CAD build for the part. Positions are in the model's coordinates, mm. Face numbers are marked on the shaded views. Round coordinates to 2 decimals unless told otherwise and drop trailing zeros. Write each loop counter-clockwise with the first axis right and the second up, starting at its lowest first coordinate (ties: lowest second). Pieces come first, ordered by that corner, then holes. Notation, with made-up numbers: (43.25, -11.5) -> (49.25, -11.5) arc R34 cw to (49.25, 23.5) -> close; hole circle Ø11 at (75.5, -37). An arc over 180 degrees is marked (long way). Answer in a Markdown table with one row per item. Add a question column.
```python
from build123d import *

# Parameters (mm, degrees)
F1_DEPTH = 11
F3_DEPTH = 1.5


with BuildPart() as f1:
    # F0 (on Top) → F1 (new body)
    with BuildSketch(Plane.XY):
        with BuildLine():
            ThreePointArc((-67.1, 20.6), (-67.312132, 20.512132), (-67.4, 20.3))
            Line((-67.4, 20.3), (-67.4, 0.3))
            ThreePointArc((-67.4, 0.3), (-67.312132, 0.087868), (-67.1, 0))
            Line((-67.1, 0), (-64.043352, 0))
            ThreePointArc((-64.043352, 0), (-63.77146, -0.173215), (-63.813539, -0.492836))
            Line((-63.813539, -0.492836), (-68.349465, -5.898542))
            ThreePointArc((-68.349465, -5.898542), (-68.41851, -6.117525), (-68.312488, -6.321192))
            Line((-68.312488, -6.321192), (-67.469839, -7.028258))
            ThreePointArc((-67.469839, -7.028258), (-67.250856, -7.097303), (-67.047189, -6.991281))
            Line((-67.047189, -6.991281), (-61.270729, -0.107164))
            ThreePointArc((-61.270729, -0.107164), (-61.167701, -0.028108), (-61.040915, 0))
            Line((-61.040915, 0), (-49.043352, 0))
            ThreePointArc((-49.043352, 0), (-48.77146, -0.173215), (-48.813539, -0.492836))
            Line((-48.813539, -0.492836), (-53.349465, -5.898542))
            ThreePointArc((-53.349465, -5.898542), (-53.41851, -6.117525), (-53.312488, -6.321192))
            Line((-53.312488, -6.321192), (-52.469839, -7.028258))
            ThreePointArc((-52.469839, -7.028258), (-52.250856, -7.097303), (-52.047189, -6.991281))
            Line((-52.047189, -6.991281), (-46.270729, -0.107164))
            ThreePointArc((-46.270729, -0.107164), (-46.167701, -0.028108), (-46.040915, 0))
            Line((-46.040915, 0), (-34.043352, 0))
            ThreePointArc((-34.043352, 0), (-33.77146, -0.173215), (-33.813539, -0.492836))
            Line((-33.813539, -0.492836), (-38.349465, -5.898542))
            ThreePointArc((-38.349465, -5.898542), (-38.41851, -6.117525), (-38.312488, -6.321192))
            Line((-38.312488, -6.321192), (-37.469839, -7.028258))
            ThreePointArc((-37.469839, -7.028258), (-37.250856, -7.097303), (-37.047189, -6.991281))
            Line((-37.047189, -6.991281), (-31.270729, -0.107164))
            ThreePointArc((-31.270729, -0.107164), (-31.167701, -0.028108), (-31.040915, 0))
            Line((-31.040915, 0), (-19.043352, 0))
            ThreePointArc((-19.043352, 0), (-18.77146, -0.173215), (-18.813539, -0.492836))
            Line((-18.813539, -0.492836), (-23.349465, -5.898542))
            ThreePointArc((-23.349465, -5.898542), (-23.41851, -6.117525), (-23.312488, -6.321192))
            Line((-23.312488, -6.321192), (-22.469839, -7.028258))
            ThreePointArc((-22.469839, -7.028258), (-22.250856, -7.097303), (-22.047189, -6.991281))
            Line((-22.047189, -6.991281), (-16.270729, -0.107164))
            ThreePointArc((-16.270729, -0.107164), (-16.167701, -0.028108), (-16.040915, 0))
            Line((-16.040915, 0), (-4.043352, 0))
            ThreePointArc((-4.043352, 0), (-3.77146, -0.173215), (-3.813539, -0.492836))
            Line((-3.813539, -0.492836), (-8.349465, -5.898542))
            ThreePointArc((-8.349465, -5.898542), (-8.41851, -6.117525), (-8.312488, -6.321192))
            Line((-8.312488, -6.321192), (-7.469839, -7.028258))
            ThreePointArc((-7.469839, -7.028258), (-7.250856, -7.097303), (-7.047189, -6.991281))
            Line((-7.047189, -6.991281), (-1.270729, -0.107164))
            ThreePointArc((-1.270729, -0.107164), (-1.167701, -0.028108), (-1.040915, 0))
            Line((-1.040915, 0), (10.956648, 0))
            ThreePointArc((10.956648, 0), (11.22854, -0.173215), (11.186461, -0.492836))
            Line((11.186461, -0.492836), (6.650535, -5.898542))
            ThreePointArc((6.650535, -5.898542), (6.58149, -6.117525), (6.687512, -6.321192))
            Line((6.687512, -6.321192), (7.530161, -7.028258))
            ThreePointArc((7.530161, -7.028258), (7.749144, -7.097303), (7.952811, -6.991281))
            Line((7.952811, -6.991281), (13.729271, -0.107164))
            ThreePointArc((13.729271, -0.107164), (13.832299, -0.028108), (13.959085, 0))
            Line((13.959085, 0), (20.524052, 0))
            ThreePointArc((20.524052, 0), (20.795944, -0.173215), (20.753865, -0.492836))
            Line((20.753865, -0.492836), (19.063644, -2.507164))
            ThreePointArc((19.063644, -2.507164), (19.021565, -2.826785), (19.293457, -3))
            Line((19.293457, -3), (21.121027, -3))
            ThreePointArc((21.121027, -3), (21.247813, -2.971892), (21.35084, -2.892836))
            Line((21.35084, -2.892836), (24.436221, 0.784177))
            ThreePointArc((24.436221, 0.784177), (24.539249, 0.863233), (24.666034, 0.891341))
            Line((24.666034, 0.891341), (25.188197, 0.891341))
            ThreePointArc((25.188197, 0.891341), (25.46009, 0.718126), (25.418011, 0.398504))
            Line((25.418011, 0.398504), (22.842019, -2.671442))
            ThreePointArc((22.842019, -2.671442), (22.813967, -2.884524), (22.995228, -3))
            Line((22.995228, -3), (25.121027, -3))
            ThreePointArc((25.121027, -3), (25.247813, -2.971892), (25.35084, -2.892836))
            Line((25.35084, -2.892836), (28.436221, 0.784177))
            ThreePointArc((28.436221, 0.784177), (28.539249, 0.863233), (28.666034, 0.891341))
            Line((28.666034, 0.891341), (29.188197, 0.891341))
            ThreePointArc((29.188197, 0.891341), (29.46009, 0.718126), (29.418011, 0.398504))
            Line((29.418011, 0.398504), (26.842019, -2.671442))
            ThreePointArc((26.842019, -2.671442), (26.813967, -2.884524), (26.995228, -3))
            Line((26.995228, -3), (29.121027, -3))
            ThreePointArc((29.121027, -3), (29.247813, -2.971892), (29.35084, -2.892836))
            Line((29.35084, -2.892836), (32.436221, 0.784177))
            ThreePointArc((32.436221, 0.784177), (32.539249, 0.863233), (32.666034, 0.891341))
            Line((32.666034, 0.891341), (33.188197, 0.891341))
            ThreePointArc((33.188197, 0.891341), (33.46009, 0.718126), (33.418011, 0.398504))
            Line((33.418011, 0.398504), (30.842019, -2.671442))
            ThreePointArc((30.842019, -2.671442), (30.813967, -2.884524), (30.995228, -3))
            Line((30.995228, -3), (33.121027, -3))
            ThreePointArc((33.121027, -3), (33.247813, -2.971892), (33.35084, -2.892836))
            Line((33.35084, -2.892836), (36.436221, 0.784177))
            ThreePointArc((36.436221, 0.784177), (36.539249, 0.863233), (36.666034, 0.891341))
            Line((36.666034, 0.891341), (37.188197, 0.891341))
            ThreePointArc((37.188197, 0.891341), (37.46009, 0.718126), (37.418011, 0.398504))
            Line((37.418011, 0.398504), (34.842019, -2.671442))
            ThreePointArc((34.842019, -2.671442), (34.813967, -2.884524), (34.995228, -3))
            Line((34.995228, -3), (37.121027, -3))
            ThreePointArc((37.121027, -3), (37.247813, -2.971892), (37.35084, -2.892836))
            Line((37.35084, -2.892836), (40.436221, 0.784177))
            ThreePointArc((40.436221, 0.784177), (40.539249, 0.863233), (40.666034, 0.891341))
            Line((40.666034, 0.891341), (41.188197, 0.891341))
            ThreePointArc((41.188197, 0.891341), (41.46009, 0.718126), (41.418011, 0.398504))
            Line((41.418011, 0.398504), (38.842019, -2.671442))
            ThreePointArc((38.842019, -2.671442), (38.813967, -2.884524), (38.995228, -3))
            Line((38.995228, -3), (41.121027, -3))
            ThreePointArc((41.121027, -3), (41.247813, -2.971892), (41.35084, -2.892836))
            Line((41.35084, -2.892836), (44.436221, 0.784177))
            ThreePointArc((44.436221, 0.784177), (44.539249, 0.863233), (44.666034, 0.891341))
            Line((44.666034, 0.891341), (45.188197, 0.891341))
            ThreePointArc((45.188197, 0.891341), (45.46009, 0.718126), (45.418011, 0.398504))
            Line((45.418011, 0.398504), (42.842019, -2.671442))
            ThreePointArc((42.842019, -2.671442), (42.813967, -2.884524), (42.995228, -3))
            Line((42.995228, -3), (46.510213, -3))
            ThreePointArc((46.510213, -3), (46.636998, -2.971892), (46.740026, -2.892836))
            Line((46.740026, -2.892836), (52.529813, 4.007164))
            ThreePointArc((52.529813, 4.007164), (52.571892, 4.326785), (52.3, 4.5))
            Line((52.3, 4.5), (46.556208, 4.5))
            ThreePointArc((46.556208, 4.5), (46.429422, 4.471892), (46.326395, 4.392836))
            Line((46.326395, 4.392836), (45.247587, 3.107164))
            ThreePointArc((45.247587, 3.107164), (45.144559, 3.028108), (45.017774, 3))
            Line((45.017774, 3), (-65.1, 3))
            ThreePointArc((-65.1, 3), (-65.312132, 3.087868), (-65.4, 3.3))
            Line((-65.4, 3.3), (-65.4, 15.3))
            ThreePointArc((-65.4, 15.3), (-65.312132, 15.512132), (-65.1, 15.6))
            Line((-65.1, 15.6), (-64.7, 15.6))
            ThreePointArc((-64.7, 15.6), (-64.487868, 15.687868), (-64.4, 15.9))
            Line((-64.4, 15.9), (-64.4, 20.3))
            ThreePointArc((-64.4, 20.3), (-64.487868, 20.512132), (-64.7, 20.6))
            Line((-64.7, 20.6), (-67.1, 20.6))
        make_face()
    extrude(amount=F1_DEPTH)

    # F2 (on face) → F3 (join)
    with BuildSketch(Plane(origin=(0, 0, 0), x_dir=(1, 0, 0), z_dir=(0, 0, -1))):
        with BuildLine():
            Line((23.684703, -3), (51.041351, -3))
            ThreePointArc((51.041351, -3), (51.313243, -2.826785), (51.271164, -2.507164))
            Line((51.271164, -2.507164), (46.740026, 2.892836))
            ThreePointArc((46.740026, 2.892836), (46.636998, 2.971892), (46.510213, 3))
            Line((46.510213, 3), (19.293457, 3))
            ThreePointArc((19.293457, 3), (19.021565, 2.826785), (19.063644, 2.507164))
            Line((19.063644, 2.507164), (23.684703, -3))
        make_face()
    extrude(amount=-F3_DEPTH)


solid = f1.part
```
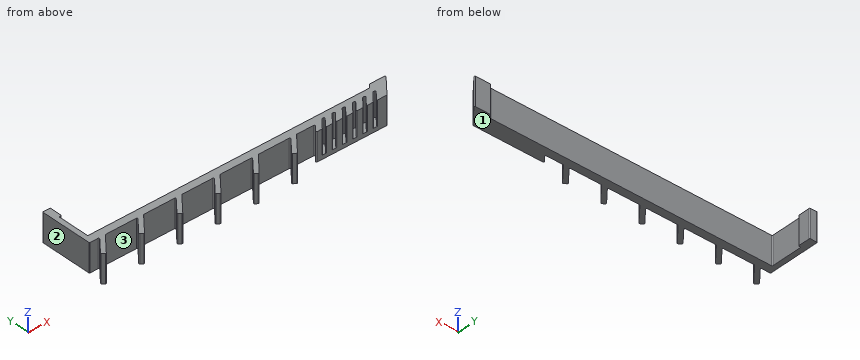
Item 1: Two-plate mould, pull along X, no slides. Class the marked faces 1, 2 and 3: +X half, -X half, draft (parallel to the pull), parting line (faces both ways), or undercut.
Item 2: Pin check, flat tips, straight feed: pin 1 (1 mm diameter, centred on x = -8, z = 6, fed in from -Y); pin 2 (1 mm diameter, centred on x = -21, z = 6.5, fed in from -Y); pin 3 (3.5 mm diameter, centred on y = 17.5, z = 3.5, fed in from +X); pin 4 (5 mm diameter, centred on x = -16, y = -2, fed in from -Z). Stop position of each tip, or through.
Item 3: Saw through at B-B on y = 7. Give the cut face in (x, z), then the cut area to 3 significant figures.
Item 4: Drill centre lines: probe 1 along X at (y, z) = (-5, 7.5); probe 2 along X at (y, z) = (-3.5, 3); probe 3 along X at (y, z) = (10, 2). Where is each one in solid material? Low to high.
Item 5: Saw through at A-A on x = -56. Give the cut face in (y, z), then the cut area to 3 significant figures.
Recorded:
| question | item | result |
|---|---|---|
| 1 | face 1 | draft |
| 1 | face 2 | -X half |
| 1 | face 3 | undercut |
| 2 | pin 1 | y = -7 |
| 2 | pin 2 | y = -6.34 |
| 2 | pin 3 | x = -64.4 |
| 2 | pin 4 | z = 0 |
| 3 | outline | (-67.4, 0) -> (-65.4, 0) -> (-65.4, 11) -> (-67.4, 11) -> close |
| 3 | area | 22.0 mm2 |
| 4 | probe 1 | -67.6 to -65.38, -52.6 to -50.38, -37.6 to -35.38, -22.6 to -20.38, -7.6 to -5.38, 7.4 to 9.62 |
| 4 | probe 2 | -66.34 to -64.12, -51.34 to -49.12, -36.34 to -34.12, -21.34 to -19.12, -6.34 to -4.12, 8.66 to 10.88 |
| 4 | probe 3 | -67.4 to -65.4 |
| 5 | outline | (0, 0) -> (3, 0) -> (3, 11) -> (0, 11) -> close |
| 5 | area | 33.0 mm2 |
